```python
from build123d import *

# Parameters (mm, degrees)
SKETCH1_W           = 101.6
SKETCH1_H           = 101.6
BOSS_EXTRUDE1_DEPTH = 3.175
SKETCH2_W           = 101.6
SKETCH2_H           = 101.6
SKETCH2_W_2         = 88.9
SKETCH2_H_2         = 88.9
BOSS_EXTRUDE2_DEPTH = 6.35
SKETCH3_R           = 0.99949
CUT_EXTRUDE1_DEPTH  = 6.35
CIRPATTERN1_COUNT   = 4
SKETCH8_W           = 88.9
SKETCH8_H           = 88.9
BOSS_EXTRUDE3_DEPTH = 1.5875
SKETCH4_W           = 101.6
SKETCH4_H           = 101.6
SKETCH4_W_2         = 95.25
SKETCH4_H_2         = 95.25
CUT_EXTRUDE2_DEPTH  = 10.525
SKETCH6_R           = 3.556
SKETCH6_R_2         = 6.096
SKETCH6_R_3         = 4.445
INPUTS_DEPTH        = 10.525
SKETCH5_R           = 0.99949
SKETCH5_W           = 27.093418
SKETCH5_H           = 18.457418
SCREEN_DEPTH        = 10.525
SKETCH7_R           = 3.556
CUT_EXTRUDE5_DEPTH  = 10.525


with BuildPart() as part:
    # Sketch1 → Boss-Extrude1 (new body)
    with BuildSketch(Plane(origin=(0, 0, 0), x_dir=(1, 0, 0), z_dir=(0, 1, 0))):
        Rectangle(SKETCH1_W, SKETCH1_H)
    extrude(amount=BOSS_EXTRUDE1_DEPTH)

    # Sketch2 → Boss-Extrude2 (add)
    with BuildSketch(Plane(origin=(0, 3.175, 0), x_dir=(1, 0, 0), z_dir=(0, 1, 0))):
        Rectangle(SKETCH2_W, SKETCH2_H)
        Rectangle(SKETCH2_W_2, SKETCH2_H_2, mode=Mode.SUBTRACT)
    extrude(amount=BOSS_EXTRUDE2_DEPTH)

    # Sketch3 → Cut-Extrude1 (cut)
    with BuildSketch(Plane.XY.offset(50.8)):
        with Locations((-38.1, 6.35)):
            Circle(SKETCH3_R)
        with Locations((38.1, 6.35)):
            Circle(SKETCH3_R)
    cut_extrude1 = extrude(amount=-CUT_EXTRUDE1_DEPTH, mode=Mode.SUBTRACT)

    # CirPattern1: Cut-Extrude1 ×4 about axis
    cirpattern1_axis = Axis((0, 10.00125, 0), (0, -1, 0))
    for i in range(1, CIRPATTERN1_COUNT):
        add(cut_extrude1.rotate(cirpattern1_axis, i * 360 / CIRPATTERN1_COUNT), mode=Mode.SUBTRACT)

    # Sketch8 → Boss-Extrude3 (add)
    with BuildSketch(Plane(origin=(0, 3.175, 0), x_dir=(1, 0, 0), z_dir=(0, 1, 0))):
        Rectangle(SKETCH8_W, SKETCH8_H)
    extrude(amount=BOSS_EXTRUDE3_DEPTH)

    # Sketch4 → Cut-Extrude2 (cut, through all)
    with BuildSketch(Plane(origin=(0, 0, 0), x_dir=(1, 0, 0), z_dir=(0, 1, 0))):
        Rectangle(SKETCH4_W, SKETCH4_H)
        Rectangle(SKETCH4_W_2, SKETCH4_H_2, mode=Mode.SUBTRACT)
    extrude(amount=CUT_EXTRUDE2_DEPTH, mode=Mode.SUBTRACT)

    # Sketch6 → Inputs (cut, through all)
    with BuildSketch(Plane.XZ):
        with Locations((0, -31.75)):
            Circle(SKETCH6_R)
        with Locations((-25.4, -31.75)):
            Circle(SKETCH6_R_2)
        with Locations((25.4, -31.75)):
            Circle(SKETCH6_R_3)
        with Locations((31.115, 25.4)):
            Circle(SKETCH6_R_2)
    extrude(amount=-INPUTS_DEPTH, mode=Mode.SUBTRACT)

    # Sketch5 → Screen (cut, through all)
    with BuildSketch(Plane.XZ):
        with Locations((-11.205633292, 14.194366708)):
            Circle(SKETCH5_R)
        with Locations((11.205633292, 14.194366708)):
            Circle(SKETCH5_R)
        with Locations((11.205633292, 36.605633292)):
            Circle(SKETCH5_R)
        with Locations((-11.205633292, 36.605633292)):
            Circle(SKETCH5_R)
        with Locations((0, 25.4)):
            Rectangle(SKETCH5_W, SKETCH5_H)
    extrude(amount=-SCREEN_DEPTH, mode=Mode.SUBTRACT)

    # Sketch7 → Cut-Extrude5 (cut, through all)
    with BuildSketch(Plane.XZ):
        with Locations((-34.925, 0)):
            Circle(SKETCH7_R)
        with Locations((34.925, 0)):
            Circle(SKETCH7_R)
    extrude(amount=-CUT_EXTRUDE5_DEPTH, mode=Mode.SUBTRACT)


solid = part.part
```
Here's how the part is built. I have some questions about the finished solid (model axes, mm). A direction names the side the tool comes from. Coordinates: 2 decimals unless noted, no trailing zeros.
1) Will these pins go through, and if not, where does the flat tip stop? pin 1 (2.5 mm diameter, centred on x = 11.21, z = 14.19, fed in from +Y); pin 2 (3 mm diameter, centred on y = 6.35, z = 38.1, fed in from +X) (3 decimals).
2) Which directions (+Z, -Z, +X, -X, +Y, -Y) give clear straight access to the entire face, cutting with the end or side of a thin tool? Please do faces 5 (the face through (-13.547, 2, 25)), 6 (the face through (-1, 7, 44.45)), 7 (the face through (-4, 9.525, 46)).
3) Imagine slicing it at A-A on z = 0. State how many separate pieces and enclosed holes the cut face has, and give its area (3 significant figures).
4) I need wall thicknesses on line 1 (Z direction, x = 30, y = 7.25) (3 decimals); line 2 (X direction, y = 1, z = 30) (3 decimals). Which ranges of each line are inside material? Lowest first, please.
5) We'd pull the mould along Z, two halves only. Please class faces 1 (the face through (-1, 5, -47.625)), 2 (the face through (-1, 7, -44.45)), 3 (the face through (47.625, 5, 1)), 4 (the face through (0, 2, 16.171)): +Z half, -Z half, draft (parallel to the pull), parting line (faces both ways), or undercut.
Response values:
1. pin 1: stops at y = 4.76
1. pin 2: stops at x = 47.625
2. face 5: +Y, -Y
2. face 6: +Y
2. face 7: +Z, -Z, +X, -X, +Y
3. separate pieces: 3
3. enclosed holes: 0
3. area: 416 mm2
4. line 1: z = -47.625 to -44.45, 44.45 to 47.625
4. line 2: x = -47.625 to -13.547, 13.547 to 27.115, 35.115 to 47.625
5. face 1: -Z half
5. face 2: undercut
5. face 3: draft
5. face 4: undercut
